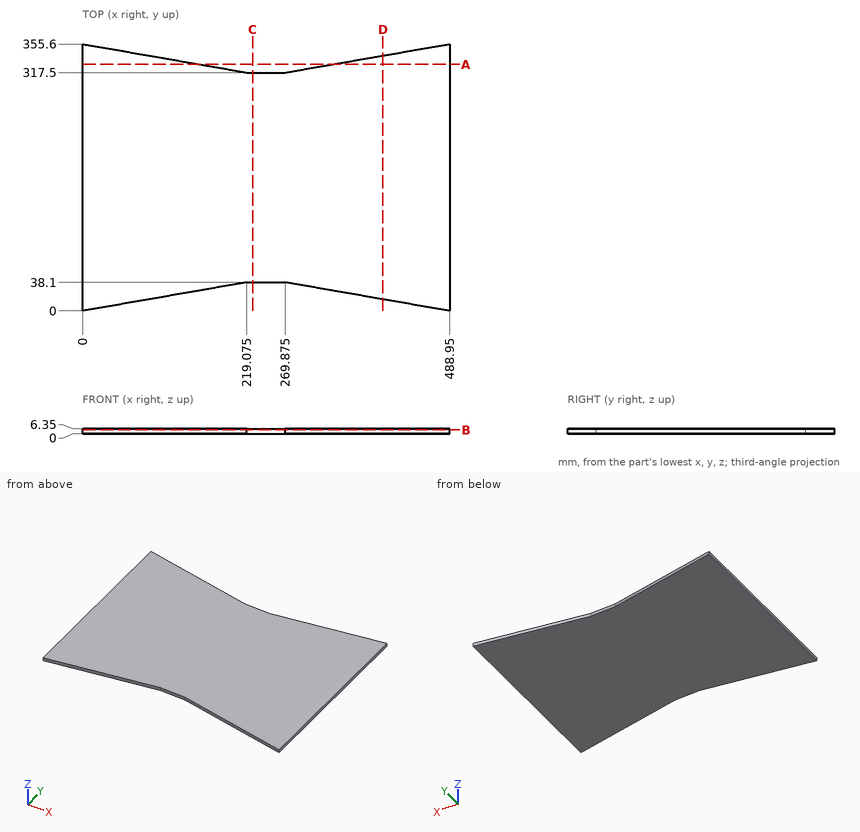
Geometry: see drawing. Coordinates: mm, zero at the bounding-box minimum. Coordinates: 2 decimals unless noted, no trailing zeros. Loops run counter-clockwise (first coordinate to the right, second up) from the corner with the lowest first, then second, coordinate; pieces in that order, holes last. Notation, with made-up numbers: (17, 84.25) - (54, 84.25) arc R32 ccw to (54, 117.25) - close; hole circle Ø10 at (74.25, -9). An arc over 180 degrees is marked (long way). Answer in a Markdown table with one row per item.
(1) Cut plane C-C on x = 226.5. Output: boundary loops of the cut face in (y, z), plus the area to 3 significant figures.
Model answer:
| item | result |
|---|---|
| outline | (38.1, 0) - (317.5, 0) - (317.5, 6.35) - (38.1, 6.35) - close |
| area | 1,770 mm² |
(2) Cut plane D-D on x = 400. Output: boundary loops of the cut face in (y, z), plus the area to 3 significant figures.
Model answer:
| item | result |
|---|---|
| outline | (15.47, 0) - (340.13, 0) - (340.13, 6.35) - (15.47, 6.35) - close |
| area | 2,060 mm² |
(3) Pin query (flat end, axial travel): P1, Ø1.9, axis at x = 250.5, z = 4, coming from the -Y side; P2, Ø1, axis at x = 91, z = 2.5, coming from the +Y side; P3, Ø3, axis at x = 253.5, z = 4.5, coming from the +Y side. Return the tip coordinate at first contact, or that it passes through.
Model answer:
| item | result |
|---|---|
| P1 | stops at y = 38.1 |
| P2 | stops at y = 339.86 |
| P3 | stops at y = 317.5 |
(4) Material intervals for L1, parallel to Y at x = 263.5, z = 2; L2, parallel to Y at x = 87, z = 4.25, sorted ascending. Write a range as from..to.
Model answer:
| item | result |
|---|---|
| L1 | y = 38.1..317.5 |
| L2 | y = 15.13..340.47 |
(5) Cut plane A-A on y = 328.5. Output: boundary loops of the cut face in (x, z) (3 decimals).
Model answer:
| item | result |
|---|---|
| outline | (0, 0) - (155.825, 0) - (155.825, 6.35) - (0, 6.35) - close; (333.125, 0) - (488.95, 0) - (488.95, 6.35) - (333.125, 6.35) - close |
(6) Cut plane B-B on z = 5. Output: boundary loops of the cut face in (x, y) (3 decimals).
Model answer:
| item | result |
|---|---|
| outline | (0, 0) - (219.075, 38.1) - (269.875, 38.1) - (488.95, 0) - (488.95, 355.6) - (269.875, 317.5) - (219.075, 317.5) - (0, 355.6) - close |
